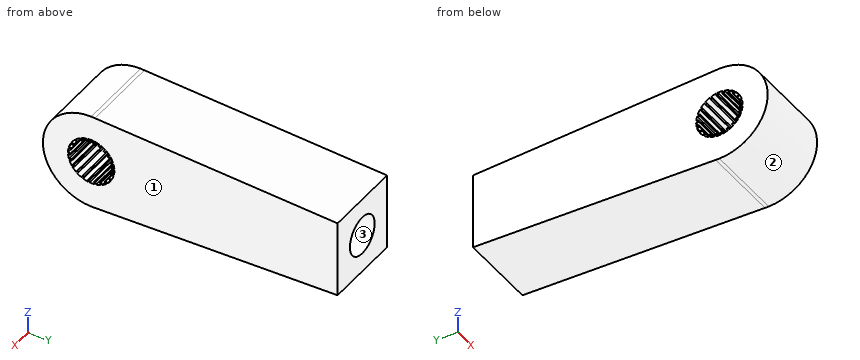
```python
from build123d import *

# Parameters (mm, degrees)
SKETCH1_R           = 6
BOSS_EXTRUDE1_DEPTH = 20
SKETCH2_R           = 5
CUT_EXTRUDE1_DEPTH  = 50
BOSS_EXTRUDE2_DEPTH = 20


with BuildPart() as part:
    # Sketch1 → Boss-Extrude1 (new body)
    with BuildSketch(Plane(origin=(0, 0, 0), x_dir=(0, 0, -1), z_dir=(1, 0, 0))):
        with BuildLine():
            Line((10, 63.75), (0, 63.75))
            Line((0, 63.75), (-10, 63.75))
            Line((-10, 63.75), (-12.461612284, 0.978886756))
            Line((-12.461612284, 0.978886756), (-12.5, 0))
            ThreePointArc((-12.5, 0), (0, -12.5), (12.5, 0))
            Line((12.5, 0), (12.461612284, 0.978886756))
            Line((12.461612284, 0.978886756), (10, 63.75))
        make_face()
        Circle(SKETCH1_R, mode=Mode.SUBTRACT)
    extrude(amount=BOSS_EXTRUDE1_DEPTH)

    # Sketch2 → Cut-Extrude1 (cut)
    with BuildSketch(Plane(origin=(0, 63.75, 0), x_dir=(1, 0, 0), z_dir=(0, 1, 0))):
        with Locations(Location((10, 0, 0), (0, 0, 270))):
            Circle(SKETCH2_R)
    extrude(amount=-CUT_EXTRUDE1_DEPTH, mode=Mode.SUBTRACT)

    # Sketch3 → Boss-Extrude2 (add)
    with BuildSketch(Plane(origin=(20, 0, 0), x_dir=(0, 0, -1), z_dir=(1, 0, 0))):
        with BuildLine():
            ThreePointArc((0, 6), (-0.214106434, 5.996178653), (-0.427940142, 5.984719478))
            Line((-0.427940142, 5.984719478), (-0.380866727, 5.326400336))
            ThreePointArc((-0.380866727, 5.326400336), (-0.190554726, 5.336599001), (0, 5.34))
            Line((0, 5.34), (0, 6))
        make_face()
        with BuildLine():
            Line((-1.504451854, 5.123692479), (-1.690395341, 5.756957842))
            ThreePointArc((-1.690395341, 5.756957842), (-1.894752362, 5.692970533), (-2.09669588, 5.621731618))
            Line((-2.09669588, 5.621731618), (-1.866059333, 5.00334114))
            ThreePointArc((-1.866059333, 5.00334114), (-1.686329602, 5.066743774), (-1.504451854, 5.123692479))
        make_face()
        with BuildLine():
            ThreePointArc((1.690395341, 5.756957842), (1.483885124, 5.813612039), (1.275484761, 5.862860959))
            Line((1.275484761, 5.862860959), (1.135181437, 5.217946254))
            ThreePointArc((1.135181437, 5.217946254), (1.320657761, 5.174114715), (1.504451853, 5.123692479))
            Line((1.504451853, 5.123692479), (1.690395341, 5.756957842))
        make_face()
        with BuildLine():
            Line((-2.887021965, 4.492293865), (-3.243844905, 5.047521197))
            ThreePointArc((-3.243844905, 5.047521197), (-3.421896722, 4.928551798), (-3.595589788, 4.803304496))
            Line((-3.595589788, 4.803304496), (-3.200074911, 4.274941001))
            ThreePointArc((-3.200074911, 4.274941001), (-3.045488083, 4.3864111), (-2.887021965, 4.492293865))
        make_face()
        with BuildLine():
            ThreePointArc((3.243844904, 5.047521197), (3.061661135, 5.160061152), (2.875577474, 5.266028313))
            Line((2.875577474, 5.266028313), (2.559263952, 4.686765198))
            ThreePointArc((2.559263952, 4.686765198), (2.72487841, 4.592454426), (2.887021965, 4.492293866))
            Line((2.887021965, 4.492293866), (3.243844904, 5.047521197))
        make_face()
        with BuildLine():
            Line((-4.035702727, 3.496956319), (-4.534497446, 3.929164403))
            ThreePointArc((-4.534497446, 3.929164403), (-4.671819361, 3.764851107), (-4.803190394, 3.59574221))
            Line((-4.803190394, 3.59574221), (-4.274839451, 3.200210567))
            ThreePointArc((-4.274839451, 3.200210567), (-4.157919231, 3.350717485), (-4.035702727, 3.496956319))
        make_face()
        with BuildLine():
            ThreePointArc((4.534497446, 3.929164404), (4.391399568, 4.0884728), (4.242708003, 4.24257337))
            Line((4.242708003, 4.24257337), (3.776010122, 3.7758903))
            ThreePointArc((3.776010122, 3.7758903), (3.908345616, 3.638740792), (4.035702727, 3.49695632))
            Line((4.035702727, 3.49695632), (4.534497446, 3.929164404))
        make_face()
        with BuildLine():
            Line((-4.857434855, 2.218316169), (-5.457791972, 2.492490078))
            ThreePointArc((-5.457791972, 2.492490078), (-5.543258979, 2.29614457), (-5.621665081, 2.096874274))
            Line((-5.621665081, 2.096874274), (-5.003281922, 1.866218104))
            ThreePointArc((-5.003281922, 1.866218104), (-4.933500492, 2.043568668), (-4.857434855, 2.218316169))
        make_face()
        with BuildLine():
            ThreePointArc((5.457791972, 2.492490078), (5.365372925, 2.685660696), (5.266119561, 2.875410365))
            Line((5.266119561, 2.875410365), (4.686846409, 2.559115225))
            ThreePointArc((4.686846409, 2.559115225), (4.775181904, 2.390238019), (4.857434855, 2.21831617))
            Line((4.857434855, 2.21831617), (5.457791972, 2.492490078))
        make_face()
        with BuildLine():
            Line((-5.2856465, 0.759961236), (-5.938928651, 0.853889029))
            ThreePointArc((-5.938928651, 0.853889029), (-5.965616722, 0.641418056), (-5.984705895, 0.428130056))
            Line((-5.984705895, 0.428130056), (-5.326388247, 0.38103575))
            ThreePointArc((-5.326388247, 0.38103575), (-5.309398883, 0.57086207), (-5.2856465, 0.759961236))
        make_face()
        with BuildLine():
            ThreePointArc((5.938928651, 0.85388903), (5.904675677, 1.065272334), (5.862901431, 1.275298713))
            Line((5.862901431, 1.275298713), (5.217982274, 1.135015855))
            ThreePointArc((5.217982274, 1.135015855), (5.255161353, 0.948092378), (5.2856465, 0.759961237))
            Line((5.2856465, 0.759961237), (5.938928651, 0.85388903))
        make_face()
        with BuildLine():
            Line((-5.2856465, -0.759961237), (-5.938928651, -0.85388903))
            ThreePointArc((-5.938928651, -0.85388903), (-5.904675677, -1.065272334), (-5.862901431, -1.275298713))
            Line((-5.862901431, -1.275298713), (-5.217982274, -1.135015855))
            ThreePointArc((-5.217982274, -1.135015855), (-5.255161353, -0.948092378), (-5.2856465, -0.759961237))
        make_face()
        with BuildLine():
            ThreePointArc((5.938928651, -0.853889029), (5.965616722, -0.641418056), (5.984705895, -0.428130056))
            Line((5.984705895, -0.428130056), (5.326388247, -0.38103575))
            ThreePointArc((5.326388247, -0.38103575), (5.309398883, -0.57086207), (5.2856465, -0.759961236))
            Line((5.2856465, -0.759961236), (5.938928651, -0.853889029))
        make_face()
        with BuildLine():
            Line((-4.857434855, -2.21831617), (-5.457791972, -2.492490078))
            ThreePointArc((-5.457791972, -2.492490078), (-5.365372925, -2.685660696), (-5.266119561, -2.875410365))
            Line((-5.266119561, -2.875410365), (-4.686846409, -2.559115225))
            ThreePointArc((-4.686846409, -2.559115225), (-4.775181904, -2.390238019), (-4.857434855, -2.21831617))
        make_face()
        with BuildLine():
            ThreePointArc((5.457791972, -2.492490078), (5.543258979, -2.29614457), (5.621665081, -2.096874274))
            Line((5.621665081, -2.096874274), (5.003281922, -1.866218104))
            ThreePointArc((5.003281922, -1.866218104), (4.933500492, -2.043568668), (4.857434855, -2.218316169))
            Line((4.857434855, -2.218316169), (5.457791972, -2.492490078))
        make_face()
        with BuildLine():
            Line((-4.035702727, -3.49695632), (-4.534497446, -3.929164404))
            ThreePointArc((-4.534497446, -3.929164404), (-4.391399568, -4.0884728), (-4.242708003, -4.24257337))
            Line((-4.242708003, -4.24257337), (-3.776010122, -3.7758903))
            ThreePointArc((-3.776010122, -3.7758903), (-3.908345616, -3.638740792), (-4.035702727, -3.49695632))
        make_face()
        with BuildLine():
            ThreePointArc((4.534497446, -3.929164403), (4.671819361, -3.764851107), (4.803190394, -3.59574221))
            Line((4.803190394, -3.59574221), (4.274839451, -3.200210567))
            ThreePointArc((4.274839451, -3.200210567), (4.157919231, -3.350717485), (4.035702727, -3.496956319))
            Line((4.035702727, -3.496956319), (4.534497446, -3.929164403))
        make_face()
        with BuildLine():
            Line((-2.887021965, -4.492293866), (-3.243844904, -5.047521197))
            ThreePointArc((-3.243844904, -5.047521197), (-3.061661135, -5.160061152), (-2.875577474, -5.266028313))
            Line((-2.875577474, -5.266028313), (-2.559263952, -4.686765198))
            ThreePointArc((-2.559263952, -4.686765198), (-2.72487841, -4.592454426), (-2.887021965, -4.492293866))
        make_face()
        with BuildLine():
            ThreePointArc((3.243844905, -5.047521197), (3.421896722, -4.928551798), (3.595589788, -4.803304496))
            Line((3.595589788, -4.803304496), (3.200074911, -4.274941001))
            ThreePointArc((3.200074911, -4.274941001), (3.045488083, -4.3864111), (2.887021965, -4.492293865))
            Line((2.887021965, -4.492293865), (3.243844905, -5.047521197))
        make_face()
        with BuildLine():
            Line((-1.504451853, -5.123692479), (-1.690395341, -5.756957842))
            ThreePointArc((-1.690395341, -5.756957842), (-1.483885124, -5.813612039), (-1.275484761, -5.862860959))
            Line((-1.275484761, -5.862860959), (-1.135181437, -5.217946254))
            ThreePointArc((-1.135181437, -5.217946254), (-1.320657761, -5.174114715), (-1.504451853, -5.123692479))
        make_face()
        with BuildLine():
            ThreePointArc((1.690395341, -5.756957842), (1.894752362, -5.692970533), (2.09669588, -5.621731618))
            Line((2.09669588, -5.621731618), (1.866059333, -5.00334114))
            ThreePointArc((1.866059333, -5.00334114), (1.686329602, -5.066743774), (1.504451854, -5.123692479))
            Line((1.504451854, -5.123692479), (1.690395341, -5.756957842))
        make_face()
        with BuildLine():
            Line((0, -5.34), (0, -6))
            ThreePointArc((0, -6), (0.214106434, -5.996178653), (0.427940142, -5.984719478))
            Line((0.427940142, -5.984719478), (0.380866727, -5.326400336))
            ThreePointArc((0.380866727, -5.326400336), (0.190554726, -5.336599001), (0, -5.34))
        make_face()
    extrude(amount=-BOSS_EXTRUDE2_DEPTH)


solid = part.part
```
Verification items for the finished model (mm, model axes). Face numbers are marked on the shaded views. Give positions to 0.01 mm unless a question says otherwise; leave off trailing zeros. Order: outer loops, then holes, each group sorted by start corner. A loop starts at its lowest first (then second) coordinate and runs counter-clockwise, first axis right, second up. Notation, with made-up numbers: (45, 1) -> (58, 1) arc R12 cw to (58, 18) -> close; hole circle Ø11 at (-35.5, -27). An arc over 180 degrees is marked (long way). Use a Markdown table: item, result.
1) Section check A-A, the plane y = 51. Record the boundary of the cut face in (x, z), then the cut area to 3 significant figures.
Results:
| item | result |
|---|---|
| outline | (0, -10.5) -> (20, -10.5) -> (20, 10.5) -> (0, 10.5) -> close; hole circle Ø10 at (10, 0) |
| area | 341 mm² |
2) Material ranges on probe 1 along X at (y, z) = (49.5, 0); probe 2 along Y at (x, z) = (14, -4); probe 3 along Y at (x, z) = (5.5, 0.25), recorded low to high.
Results:
| item | result |
|---|---|
| probe 1 | 0 to 5, 15 to 20 |
| probe 2 | -11.84 to -4.47, 3.54 to 4, 4.47 to 63.75 |
| probe 3 | -12.5 to -5.99, 5.33 to 13.75 |
3) Mould release check, pull along Z, two halves, no side actions. Record for the marked faces 1, 2 and 3: pulls with the +Z half, pulls with the -Z half, needs draft (parallel to the pull), parting line crosses it, or undercut.
Results:
| item | result |
|---|---|
| face 1 | needs draft |
| face 2 | parting line crosses it |
| face 3 | undercut |
4) Section check B-B, the plane z = 8.25. Record the boundary of the cut face in (x, y), then the cut area to 3 significant figures.
Results:
| item | result |
|---|---|
| outline | (0, -9.39) -> (20, -9.39) -> (20, 63.75) -> (0, 63.75) -> close |
| area | 1,460 mm² |
5) Section check D-D, the plane z = -8.5. Record the boundary of the cut face in (x, y), then the cut area to 3 significant figures.
Results:
| item | result |
|---|---|
| outline | (0, -9.17) -> (20, -9.17) -> (20, 63.75) -> (0, 63.75) -> close |
| area | 1,460 mm² |
6) Section check C-C, the plane y = 20.5. Record the boundary of the cut face in (x, z).
Results:
| item | result |
|---|---|
| outline | (0, -11.7) -> (20, -11.7) -> (20, 11.7) -> (0, 11.7) -> close; hole circle Ø10 at (10, 0) |
7) Depth check by flat-ended pin: pin 1 Ø12 at (x, y) = (16.5, 47) entering from +Z; pin 2 Ø0.7 at (x, y) = (5.5, 5.5) entering from -Z; pin 3 Ø1.5 at (x, z) = (10.5, -9) entering from -Y. Enter the tip coordinate at first touch or a pass-through.
Results:
| item | result |
|---|---|
| pin 1 | z = 10.89 |
| pin 2 | z = -12.3 |
| pin 3 | y = -9.39 |
